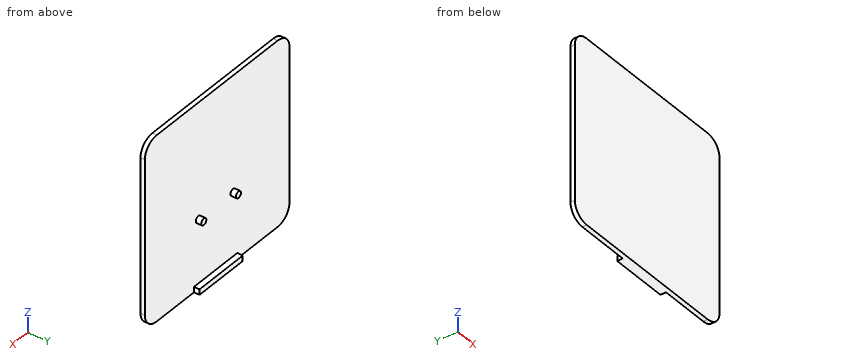
from build123d import *

# Parameters (mm, degrees)
BOSS_EXTRUDE1_DEPTH = 2
SKETCH2_R           = 1.5
SKETCH2_W           = 25.4
SKETCH2_H           = 2.5
BOSS_EXTRUDE2_DEPTH = 2.5


with BuildPart() as part:
    # Sketch1 → Boss-Extrude1 (new body)
    with BuildSketch(Plane(origin=(0, 0, 0), x_dir=(1, 0, 0), z_dir=(0, 1, 0))):
        with BuildLine():
            Line((-35.892490242, -26.522279469), (35.107509758, -26.522279469))
            ThreePointArc((35.107509758, -26.522279469), (40.057257226, -24.472026937), (42.107509758, -19.522279469))
            Line((42.107509758, -19.522279469), (42.107509758, 51.477720531))
            ThreePointArc((42.107509758, 51.477720531), (40.057257226, 56.427467999), (35.107509758, 58.477720531))
            Line((35.107509758, 58.477720531), (-35.892490242, 58.477720531))
            ThreePointArc((-35.892490242, 58.477720531), (-40.84223771, 56.427467999), (-42.892490242, 51.477720531))
            Line((-42.892490242, 51.477720531), (-42.892490242, -19.522279469))
            ThreePointArc((-42.892490242, -19.522279469), (-40.84223771, -24.472026937), (-35.892490242, -26.522279469))
        make_face()
    extrude(amount=BOSS_EXTRUDE1_DEPTH)

    # Sketch2 → Boss-Extrude2 (add)
    with BuildSketch(Plane(origin=(0, 2, 0), x_dir=(1, 0, 0), z_dir=(0, 1, 0))):
        with Locations(Location((-9.711578579, 26.678960322, 0), (0, 0, 90))):
            Circle(SKETCH2_R)
        with Locations(Location((10.688421421, 26.678960322, 0), (0, 0, 90))):
            Circle(SKETCH2_R)
        with Locations((0.488421421, 57.227720531)):
            Rectangle(SKETCH2_W, SKETCH2_H)
    extrude(amount=BOSS_EXTRUDE2_DEPTH)


solid = part.part
Verification items for the finished model (mm, model axes). Coordinates: 2 decimals unless noted, no trailing zeros. Loops run counter-clockwise (first coordinate to the right, second up) from the corner with the lowest first, then second, coordinate; pieces in that order, holes last. Notation, with made-up numbers: M 48.5,-12 L 63.5,-12 A31 cw 63.5,26 Z; hole C 12.5,-8 d1. An arc over 180 degrees is marked long. One line per item, written item: value.
1. Section check D-D on x = 20. Record the cut outline in (y, z).
Answers follow:
outline: M 0,-58.48 L 2,-58.48 L 2,26.52 L 0,26.52 Z
2. Section check C-C on z = -7. Record the cut outline in (x, y), plus the area to 3 significant figures.
Answers follow:
outline: M -42.89,0 L 42.11,0 L 42.11,2 L -42.89,2 Z
area: 170 mm^2
3. Material ranges on line 1 along Y through (x, z) = (1, -13); line 2 along Z through (x, y) = (-1.5, 2.75); line 3 along X through (y, z) = (1.5, 23.5), recorded low to high. Write a range as from..to.
Answers follow:
line 1: 0..2
line 2: -58.48..-55.98
line 3: -41.65..40.87
4. Section check A-A on y = 3.5. Record the cut outline in (x, z).
Answers follow:
outline: M -12.21,-58.48 L 13.19,-58.48 L 13.19,-55.98 L -12.21,-55.98 Z; C -9.71,-26.68 d3; C 10.69,-26.68 d3
5. Gauge pin test, flat ends, axial feed: P1, Ø1, axis at x = 17.5, z = -17.5, coming from the +Y side; P2, Ø2, axis at y = 3.5, z = -57, coming from the -X side; P3, Ø0.8, axis at y = 3.5, z = -57.5, coming from the +X side. Record the tip position at first contact, or that the pin passes through.
Answers follow:
P1: y = 2
P2: x = -12.21
P3: x = 13.19
6. Section check B-B on x = 2.5. Record the cut outline in (y, z).
Answers follow:
outline: M 0,-58.48 L 4.5,-58.48 L 4.5,-55.98 L 2,-55.98 L 2,26.52 L 0,26.52 Z
